Source: CAD feature listing. Evaluate the final solid. Frame: model axes, mm. A direction names the side the tool comes from. Round coordinates to 2 decimals unless told otherwise and drop trailing zeros. Loops run counter-clockwise (first coordinate to the right, second up) from the corner with the lowest first, then second, coordinate; pieces in that order, holes last. Notation, with made-up numbers: (40, 42.5) - (61, 42.5) arc R9 ccw to (61, 57.5) - close; hole circle Ø2 at (-31, 39.5). An arc over 180 degrees is marked (long way). One line per question, with ' | ' between items.
from build123d import *

# Parameters (mm, degrees)
SKETCH1_R           = 1.19126
BOSS_EXTRUDE1_DEPTH = 11.1125
SKETCH4_W           = 3.175
SKETCH4_H           = 0.39751
CUT_EXTRUDE1_START  = -2.38252
SKETCH6_R           = 0.39751
CUT_EXTRUDE1_DEPTH  = 11.1125


with BuildPart() as part:
    # Sketch1 → Boss-Extrude1 (new body)
    with BuildSketch(Plane.XY):
        Circle(SKETCH1_R)
    extrude(amount=-BOSS_EXTRUDE1_DEPTH)

    # Sketch2 → Cut-Revolve1 (revolve, cut)
    with BuildSketch(Plane(origin=(0, 0, 0), x_dir=(0, 0, -1), z_dir=(1, 0, 0))):
        Polygon((0, 0.39751), (1.5875, 1.19126), (0, 1.19126), align=None)
    revolve(axis=Axis((0, 0, 0), (0, 0, -1)), mode=Mode.SUBTRACT)

    # Sketch4 → Cut-Revolve2 (revolve, cut)
    with BuildSketch(Plane(origin=(0, 0, 0), x_dir=(0, 0, -1), z_dir=(1, 0, 0))):
        with Locations((9.525, 0.992505)):
            Rectangle(SKETCH4_W, SKETCH4_H)
    revolve(axis=Axis((0, 0, 0), (0, 0, -1)), mode=Mode.SUBTRACT)

    # Sketch5 → Cut-Revolve3 (revolve, cut)
    with BuildSketch(Plane(origin=(0, 0, 0), x_dir=(0, 0, -1), z_dir=(1, 0, 0))):
        Polygon((0, 0.39751), (1.5875, 0.19812), (1.5875, 0), (0, 0), align=None)
    revolve(axis=Axis((0, 0, 0), (0, 0, -1)), mode=Mode.SUBTRACT)

    # Sketch6 → Cut-Extrude1 (cut)
    with BuildSketch(Plane.XY.offset(CUT_EXTRUDE1_START)):
        Circle(SKETCH6_R)
    extrude(amount=-CUT_EXTRUDE1_DEPTH, mode=Mode.SUBTRACT)

    # Sketch7 → Cut-Revolve4 (revolve, cut)
    with BuildSketch(Plane(origin=(0, 0, 0), x_dir=(0, 0, -1), z_dir=(1, 0, 0))):
        Polygon((1.5875, 0.19812), (2.38252, 0.39751), (2.38252, 0), (1.5875, 0), align=None)
    revolve(axis=Axis((0, 0, 0), (0, 0, -1)), mode=Mode.SUBTRACT)


solid = part.part
1. Section query A-A, the plane y = 0. Return loops of the section in (x, z).
Worked out:
outline: (-1.19, -7.94) - (-0.79, -7.94) - (-0.79, -11.11) - (-0.4, -11.11) - (-0.4, -2.38) - (-0.2, -1.59) - (-0.4, 0) - (-1.19, -1.59) - close; (0.2, -1.59) - (0.4, -2.38) - (0.4, -11.11) - (0.79, -11.11) - (0.79, -7.94) - (1.19, -7.94) - (1.19, -1.59) - (0.4, 0) - close
2. Access query for faces 1 (the cylindrical face through (1.136, 0.358, -4.718)), 2 (the flat face through (-1, 0, -7.938)). Directions: +Z, -Z, +X, -X, +Y, -Y. A direction counts if a zero-diameter tool reaches every point of the face in a straight line with its end or side. Return the directions, or none.
Worked out:
face 1: +Z, -Z | face 2: -Z
3. Material intervals for probe 1 along Y at (x, z) = (0, -7); probe 2 along X at (y, z) = (0, -8.5); probe 3 along Y at (x, z) = (0.05, -0.75), sorted ascending.
Worked out:
probe 1: y = -1.19 to -0.4, 0.4 to 1.19 | probe 2: x = -0.79 to -0.4, 0.4 to 0.79 | probe 3: y = -0.77 to -0.3, 0.3 to 0.77
4. Section query C-C, the plane z = -4.25. Return loops of the section in (x, y).
Worked out:
outline: circle Ø2.38 at (0, 0); hole circle Ø0.8 at (0, 0)
